Job drawing, mm, ordinate dimensions from the low corner. One solid piece. Round coordinates to 2 decimals unless told otherwise and drop trailing zeros. Loops run counter-clockwise (first coordinate to the right, second up) from the corner with the lowest first, then second, coordinate; pieces in that order, holes last.
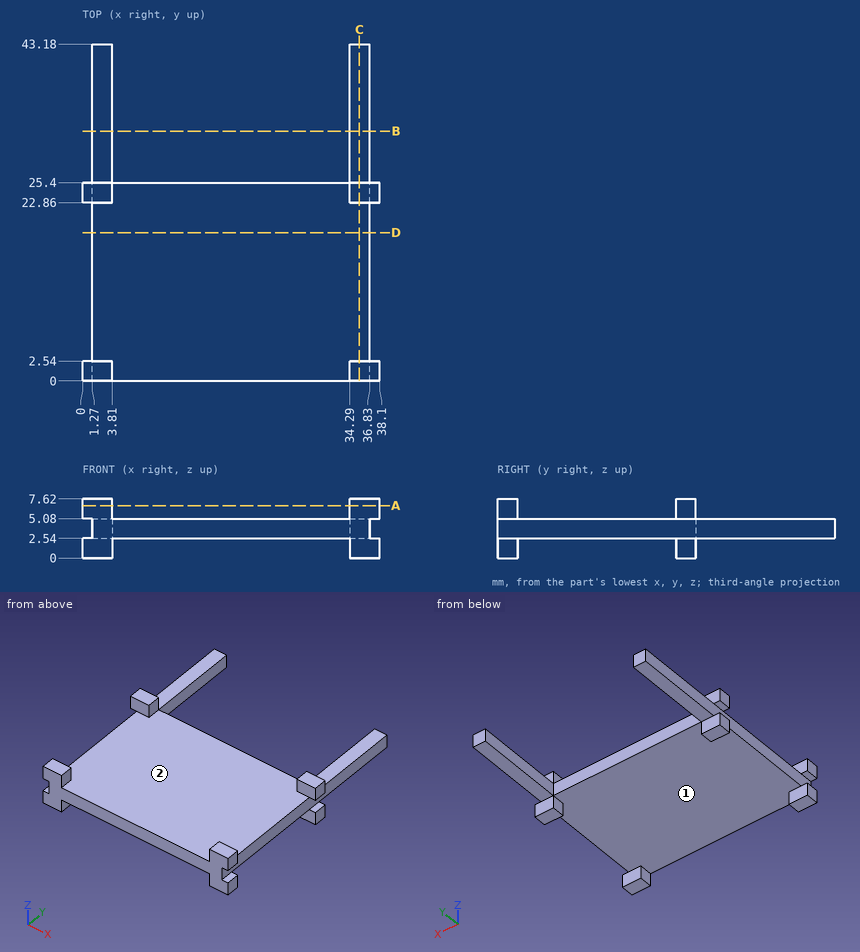
Item 1: Probe line 1 (Y direction, x = 35.5, z = 7.25); line 2 (X direction, y = 39, z = 3.25); line 3 (Z direction, x = 14, y = 21). List the from-to ranges inside material, lowest first.
Answers follow:
line 1: y = 0 to 2.54, 22.86 to 25.4
line 2: x = 1.27 to 3.81, 34.29 to 36.83
line 3: z = 2.54 to 5.08
Item 2: Two-plate mould, pull along X, no slides. Class the marked faces 1 and 2: released by +X, released by -X, zero draft, split by the parting line, or undercut.
Answers follow:
face 1: undercut
face 2: undercut
Item 3: Cut at C-C, the plane x = 35.5. Give the cut face in (y, z).
Answers follow:
outline: (0, 0) - (2.54, 0) - (2.54, 2.54) - (22.86, 2.54) - (22.86, 0) - (25.4, 0) - (25.4, 2.54) - (43.18, 2.54) - (43.18, 5.08) - (25.4, 5.08) - (25.4, 7.62) - (22.86, 7.62) - (22.86, 5.08) - (2.54, 5.08) - (2.54, 7.62) - (0, 7.62) - close
Item 4: Cut at B-B, the plane y = 32. Give the cut face in (x, z).
Answers follow:
outline: (1.27, 2.54) - (3.81, 2.54) - (3.81, 5.08) - (1.27, 5.08) - close; (34.29, 2.54) - (36.83, 2.54) - (36.83, 5.08) - (34.29, 5.08) - close
Item 5: Flat gauge pins, fed straight in: P1, Ø1, axis at x = 20.5, z = 3.5, coming from the +Y side; P2, Ø2, axis at y = 26.5, z = 4, coming from the -X side; P3, Ø2, axis at y = 25.5, z = 5, coming from the +X side; P4, Ø5, axis at x = 34, y = 32, coming from the -Z side. Where does each tip first touch, or does it go through?
Answers follow:
P1: stops at y = 25.4
P2: stops at x = 1.27
P3: stops at x = 38.1
P4: stops at z = 2.54
Item 6: Cut at D-D, the plane y = 19. Give the cut face in (x, z), plus the area to 3 significant figures.
Answers follow:
outline: (1.27, 2.54) - (36.83, 2.54) - (36.83, 5.08) - (1.27, 5.08) - close
area: 90.3 mm2
Item 7: Cut at A-A, the plane z = 6.75. Give the cut face in (x, y).
Answers follow:
outline: (0, 0) - (3.81, 0) - (3.81, 2.54) - (0, 2.54) - close; (0, 22.86) - (3.81, 22.86) - (3.81, 25.4) - (0, 25.4) - close; (34.29, 0) - (38.1, 0) - (38.1, 2.54) - (34.29, 2.54) - close; (34.29, 22.86) - (38.1, 22.86) - (38.1, 25.4) - (34.29, 25.4) - close
